from build123d import *

# Parameters (mm, degrees)
SKETCH1_W           = 305
SKETCH1_H           = 305
BOSS_EXTRUDE1_DEPTH = 0.5
BOSS_EXTRUDE2_DEPTH = 0.5
FILLET1_R           = 1
FILLET2_R           = 1.5
FILLET3_R           = 3


with BuildPart() as part:
    # Sketch1 → Boss-Extrude1 (new body)
    with BuildSketch(Plane(origin=(0, 0, 0), x_dir=(1, 0, 0), z_dir=(0, 1, 0))):
        Rectangle(SKETCH1_W, SKETCH1_H)
    extrude(amount=BOSS_EXTRUDE1_DEPTH)

    # Sketch2 → Boss-Extrude2 (add)
    with BuildSketch(Plane(origin=(0, 0.5, 0), x_dir=(1, 0, 0), z_dir=(0, 1, 0))):
        Polygon((-72.5, -152.5), (-122.5, -152.5), (-112.5, -162.5), (-82.5, -162.5), align=None)
        Polygon((112.5, -162.5), (122.5, -152.5), (72.5, -152.5), (82.5, -162.5), align=None)
        Polygon((-144.901923792, 155.5), (-146.6339746, 152.5), (146.6339746, 152.5), (144.901923792, 155.5), align=None)
    extrude(amount=-BOSS_EXTRUDE2_DEPTH)

    # Fillet1
    fillet1_edges = [part.edges().sort_by_distance(p)[0] for p in [
        (-144.901923792, 0.25, -155.5),
        (144.901923792, 0.25, -155.5),
        (152.5, 0.25, 152.5),
        (-152.5, 0.25, 152.5),
        (-152.5, 0.25, -152.5),
        (152.5, 0.25, -152.5),
    ]]
    fillet(fillet1_edges, radius=FILLET1_R)

    # Fillet2
    fillet2_edges = [part.edges().sort_by_distance(p)[0] for p in [
        (-146.6339746, 0.25, -152.5),
        (146.6339746, 0.25, -152.5),
    ]]
    fillet(fillet2_edges, radius=FILLET2_R)

    # Fillet3
    fillet3_edges = [part.edges().sort_by_distance(p)[0] for p in [
        (-72.5, 0.25, 152.5),
        (-82.5, 0.25, 162.5),
        (-112.5, 0.25, 162.5),
        (122.5, 0.25, 152.5),
        (112.5, 0.25, 162.5),
        (82.5, 0.25, 162.5),
        (72.5, 0.25, 152.5),
        (-122.5, 0.25, 152.5),
    ]]
    fillet(fillet3_edges, radius=FILLET3_R)


solid = part.part
Could you check a few things on this model? Use its own coordinates, in mm. A direction names the side the tool comes from. Round coordinates to 2 decimals unless told otherwise and drop trailing zeros. Order: outer loops, then holes, each group sorted by start corner. A loop starts at its lowest first (then second) coordinate and runs counter-clockwise, first axis right, second up. Notation, with made-up numbers: M 65,-1 L 109,-1 A24 ccw 109,24 Z; hole C 45.5,54 d6. An arc over 180 degrees is marked long. One line per item, written item: value.
(1) I need wall thicknesses on line 1 along Z through (x, y) = (52, 0.1); line 2 along Z through (x, y) = (-73, 0.45). Which ranges of each line are inside material? Lowest first, please. Write a range as from..to.
Ans:
line 1: z = -155.5..152.5
line 2: z = -155.5..153.06
(2) Imagine slicing it at B-B (x = -49.5). Write out the boundary of the cut face in (y, z), and give its area (3 significant figures).
Ans:
outline: M 0,-155.5 L 0.5,-155.5 L 0.5,152.5 L 0,152.5 Z
area: 154 mm^2
(3) If we mould it in two halves opening along X, with no side actions, what happens to faces 1 (the flat face through (-77.6, 0.3, 157.6)), 2 (the flat face through (-117.6, 0.3, 157.4)), 3 (the flat face through (-2, 0, 1))? For each: released by +X, released by -X, zero draft, split by the parting line, or undercut.
Ans:
face 1: undercut
face 2: released by -X
face 3: zero draft
(4) Which directions (+Z, -Z, +X, -X, +Y, -Y) give clear straight access to the entire face, cutting with the end or side of a thin tool? Please do faces 4 (the flat face through (-2, 0.5, 1)), 5 (the flat face through (77.4, 0.3, 157.4)).
Ans:
face 4: +Z, -Z, +X, -X, +Y
face 5: +Z, +Y, -Y
